Study the drawing (mm; zero at the part's minimum x, y, z) and answer. A direction names the side the tool comes from. Coordinates: 2 decimals unless noted, no trailing zeros. Order: outer loops, then holes, each group sorted by start corner. A loop starts at its lowest first (then second) coordinate and runs counter-clockwise, first axis right, second up. Notation, with made-up numbers: M 4.25,-14.75 L 30.25,-14.75 A10 cw 30.25,-6.75 Z; hole C -38.75,26.25 d8. An arc over 180 degrees is marked long. Use a Markdown table: item, result. Add a question column.
1) Find the intervals of material crossed by probe 1 along X at (y, z) = (16.5, 1.75) (1 decimal); probe 2 along X at (y, z) = (29, 2.25) (1 decimal); probe 3 along Z at (x, y) = (28.5, 16), in increasing order. Write a range as [from, to].
2) Each of these flat-tipped pins is pushed along its axis until it touches: pin 1 Ø2.5 at (y, z) = (21.5, 7.5) entering from -X; pin 2 Ø6 at (y, z) = (17, 9) entering from +X; pin 3 Ø10 at (x, y) = (10.36, 4.83) entering from +Z. Where does it stop, or does it pass through?
3) Find section D-D on z = 8. Write down the section's boundary in (x, y).
4) Find section A-A on z = 1.5. Count the separate pieces of the cut face and the enclosed holes in it, plus the area to 3 significant figures.
5) Find section B-B on y = 15. Write down the section's boundary in (x, z) (1 decimal), plus the area to 3 significant figures.
6) For the marked faces 1, 2 and 3, determine the directions among +Z, -Z, +X, -X, +Y, -Y from which every point of the face is accessible in a straight line to the end or side of a thin tool.
7) Find section C-C on x = 55. Write down the section's boundary in (y, z).
8) The mould has two halves that part along Y. Classify the marked faces 4, 5 and 6: released by +Y, released by -Y, zero draft, split by the parting line, or undercut.
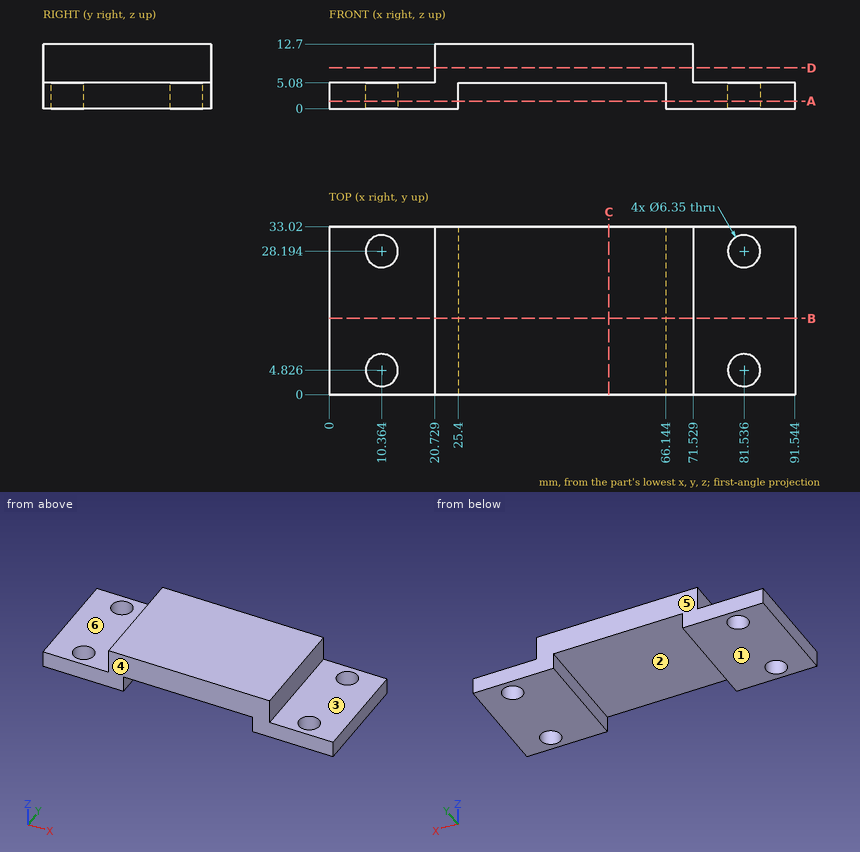
Check result:
| question | item | result |
|---|---|---|
| 1 | probe 1 | x = [0, 25.4], [66.1, 91.5] |
| 1 | probe 2 | x = [0, 7.3], [13.4, 25.4], [66.1, 78.5], [84.6, 91.5] |
| 1 | probe 3 | z = [5.08, 12.7] |
| 2 | pin 1 | stops at x = 20.73 |
| 2 | pin 2 | stops at x = 71.53 |
| 2 | pin 3 | stops at z = 5.08 |
| 3 | outline | M 20.73,0 L 71.53,0 L 71.53,33.02 L 20.73,33.02 Z |
| 4 | separate pieces | 2 |
| 4 | enclosed holes | 4 |
| 4 | area | 1,550 mm2 |
| 5 | outline | M 0,0 L 25.4,0 L 25.4,5.1 L 66.1,5.1 L 66.1,0 L 91.5,0 L 91.5,5.1 L 71.5,5.1 L 71.5,12.7 L 20.7,12.7 L 20.7,5.1 L 0,5.1 Z |
| 5 | area | 645 mm2 |
| 6 | face 1 | -Z, +X, -X, +Y, -Y |
| 6 | face 2 | -Z, +Y, -Y |
| 6 | face 3 | +Z, +X, +Y, -Y |
| 7 | outline | M 0,5.08 L 33.02,5.08 L 33.02,12.7 L 0,12.7 Z |
| 8 | face 4 | released by -Y |
| 8 | face 5 | released by +Y |
| 8 | face 6 | zero draft |
